CAD build for the part. Positions are in the model's coordinates, mm. A direction names the side the tool comes from. Round coordinates to 2 decimals unless told otherwise and drop trailing zeros. Loops run counter-clockwise (first coordinate to the right, second up) from the corner with the lowest first, then second, coordinate; pieces in that order, holes last.
from build123d import *

# Parameters (mm, degrees)
SKETCH1_R                = 4.25
BOSS_EXTRUDE1_DEPTH      = 4
BOSS_EXTRUDE2_DEPTH      = 4
SKETCH3_R                = 2
BOSS_EXTRUDE3_DEPTH      = 2
BOSS_EXTRUDE4_DEPTH      = 53.7
BOSS_EXTRUDE4_DEPTH_BACK = 4
CUT_EXTRUDE1_DEPTH       = 53.7
BOSS_EXTRUDE5_DEPTH      = 120
CUT_EXTRUDE2_DEPTH       = 120
CUT_EXTRUDE2_DEPTH_BACK  = 120
BOSS_EXTRUDE6_DEPTH      = 53.7
BOSS_EXTRUDE6_DEPTH_BACK = 4
CUT_EXTRUDE3_DEPTH       = 53.7
CUT_EXTRUDE4_DEPTH       = 53.7
SKETCH18_W               = 12.575700543
SKETCH18_H               = 12.198178211
CUT_EXTRUDE9_DEPTH       = 98.7
BOSS_EXTRUDE7_DEPTH      = 20
CUT_EXTRUDE11_DEPTH      = 20
SKETCH22_R               = 3
CUT_EXTRUDE12_DEPTH      = 10
CUT_EXTRUDE13_DEPTH      = 99
CUT_EXTRUDE14_DEPTH      = 99
BOSS_EXTRUDE8_DEPTH      = 12


with BuildPart() as part:
    # Sketch1 → Boss-Extrude1 (new body)
    with BuildSketch(Plane.XY):
        Polygon((0, 10), (0, -15), (-30, -35), (-30, 10), (-15, 25), align=None)
        with Locations((-15, 10)):
            Circle(SKETCH1_R, mode=Mode.SUBTRACT)
    extrude(amount=BOSS_EXTRUDE1_DEPTH)



with BuildPart() as body_2:
    # Sketch2 → Boss-Extrude2 (new body)
    with BuildSketch(Plane.XY.offset(-49.7)):
        Polygon((-30, -35), (-30, 10), (-15, 25), (0, 10), (0, -15), align=None)
    extrude(amount=-BOSS_EXTRUDE2_DEPTH)

    # Sketch3 → Boss-Extrude3 (add)
    with BuildSketch(Plane.XY.offset(-49.7)):
        with Locations((-15, 10)):
            Circle(SKETCH3_R)
    extrude(amount=BOSS_EXTRUDE3_DEPTH)


with BuildPart() as part_1:
    add(part.part)

    add(body_2.part)  # Boss-Extrude4 merges body 2
    # Sketch4 → Boss-Extrude4 (add, two sides: drawn at the far end of the back side and taken through both)
    with BuildSketch(Plane.XY.offset(-49.7).offset(-BOSS_EXTRUDE4_DEPTH_BACK)):
        Polygon((-30, -35), (0, -35), (0, -15), align=None)
    extrude(amount=BOSS_EXTRUDE4_DEPTH + BOSS_EXTRUDE4_DEPTH_BACK)

    # Sketch5 → Cut-Extrude1 (cut)
    with BuildSketch(Plane(origin=(0, 0, 0), x_dir=(0, 0, -1), z_dir=(1, 0, 0))):
        Polygon((24.85, -15), (49.7, -15), (49.7, -35), (0, -35), (0, -15), align=None)
    extrude(amount=-CUT_EXTRUDE1_DEPTH, mode=Mode.SUBTRACT)


with BuildPart() as cut_extrude1_piece_1:
    # of the separate pieces the step leaves, piece 1, a body of its own (cut_extrude1_pieces)
    add(part_1.part.solids().sort_by_distance((-30, -35, -49.7))[0])



with BuildPart() as cut_extrude1_piece_2:
    # of the separate pieces the step leaves, piece 2, a body of its own (cut_extrude1_pieces)
    add(part_1.part.solids().sort_by_distance((0, -35, 0))[0])


with BuildPart() as cut_extrude1_piece_1_1:
    add(cut_extrude1_piece_1.part)

    add(cut_extrude1_piece_2.part)  # Boss-Extrude5 merges Cut-Extrude1 piece 2
    # Sketch6 → Boss-Extrude5 (add)
    with BuildSketch(Plane(origin=(0, 0, 0), x_dir=(0, 0, -1), z_dir=(1, 0, 0))):
        Polygon((0, -35), (-4, -35), (24.85, -46.609657949), (53.7, -35), (49.7, -35), (24.85, -45), align=None)
    extrude(amount=-BOSS_EXTRUDE5_DEPTH)

    # Sketch7 → Cut-Extrude2 (cut, two sides: drawn at the far end of the back side and taken through both)
    with BuildSketch(Plane.XY.offset(-49.7).offset(-CUT_EXTRUDE2_DEPTH_BACK)):
        Polygon((-30, -35), (-120, -35), (-120, -46.609657949), align=None)
    extrude(amount=CUT_EXTRUDE2_DEPTH + CUT_EXTRUDE2_DEPTH_BACK, mode=Mode.SUBTRACT)

    # Sketch8 → Boss-Extrude6 (add, two sides: drawn at the far end of the back side and taken through both)
    with BuildSketch(Plane.XY.offset(-49.7).offset(-BOSS_EXTRUDE6_DEPTH_BACK)):
        Polygon((-30, -35), (-30, -12.5), (-120, -46.609657949), align=None)
    extrude(amount=BOSS_EXTRUDE6_DEPTH + BOSS_EXTRUDE6_DEPTH_BACK)

    # Sketch9 → Cut-Extrude3 (cut)
    with BuildSketch(Plane(origin=(3.949939329, -30.620586856, 0), x_dir=(0.991782404932817, 0.12793616089940293, 0), z_dir=(0.12793616089940293, -0.991782404932817, 0))):
        Polygon((-124.976949291, -24.85), (-34.231237779, -53.7), (-124.976949291, -53.7), align=None)
    extrude(amount=-CUT_EXTRUDE3_DEPTH, mode=Mode.SUBTRACT)

    # Sketch10 → Cut-Extrude4 (cut)
    with BuildSketch(Plane(origin=(3.949939329, -30.620586856, 0), x_dir=(0.991782404932817, 0.12793616089940293, 0), z_dir=(0.12793616089940293, -0.991782404932817, 0))):
        Polygon((-124.976949291, -24.85), (-34.231237779, 4), (-124.976949291, 4), align=None)
    extrude(amount=-CUT_EXTRUDE4_DEPTH, mode=Mode.SUBTRACT)

    # Sketch18 → Cut-Extrude9 (cut)
    with BuildSketch(Plane(origin=(-100, 0, 0), x_dir=(0, 0, -1), z_dir=(1, 0, 0))):
        with Locations((24.80300407, -45.072632523)):
            Rectangle(SKETCH18_W, SKETCH18_H)
    extrude(amount=-CUT_EXTRUDE9_DEPTH, mode=Mode.SUBTRACT)

    # Sketch19 → Boss-Extrude7 (add)
    with BuildSketch(Plane.ZY.offset(100)):
        Polygon((-31.090854341, -39.02973396), (-31.090854341, -44.098247751), (-24.85, -46.609657949), (-18.515153798, -44.060424064), (-18.515153798, -39.02973396), align=None)
    extrude(amount=BOSS_EXTRUDE7_DEPTH)

    # Sketch20 → Cut-Extrude11 (cut)
    with BuildSketch(Plane.ZY.offset(120)):
        with BuildLine():
            Line((-18.515153798, -39.02973396), (-24.80300407, -39.02973396))
            Line((-24.80300407, -39.02973396), (-24.804747468, -39.310924888))
            ThreePointArc((-24.804747468, -39.310924888), (-22.337699017, -40.346275812), (-21.317663529, -42.819695955))
            ThreePointArc((-21.317663529, -42.819695955), (-21.889089638, -44.738955206), (-23.417250653, -46.033098856))
            Line((-23.417250653, -46.033098856), (-18.515153798, -44.060424064))
            Line((-18.515153798, -44.060424064), (-18.515153798, -39.02973396))
        make_face()
        with BuildLine():
            Line((-24.804747468, -39.310924888), (-24.80300407, -39.02973396))
            Line((-24.80300407, -39.02973396), (-31.090854341, -39.02973396))
            Line((-31.090854341, -39.02973396), (-31.090854341, -44.098247751))
            Line((-31.090854341, -44.098247751), (-24.85, -46.609657949))
            Line((-24.85, -46.609657949), (-24.848256601, -46.328467021))
            ThreePointArc((-24.848256601, -46.328467021), (-28.335273102, -42.797941388), (-24.804747468, -39.310924888))
        make_face()
        with BuildLine():
            ThreePointArc((-23.617143522, -46.113538642), (-24.223054162, -46.276254695), (-24.848256601, -46.328467021))
            Line((-24.848256601, -46.328467021), (-24.85, -46.609657949))
            Line((-24.85, -46.609657949), (-23.617143522, -46.113538642))
        make_face()
    extrude(amount=-CUT_EXTRUDE11_DEPTH, mode=Mode.SUBTRACT)

    # Sketch22 → Cut-Extrude12 (cut)
    with BuildSketch(Plane.ZY.offset(120)):
        with Locations((-24.826502035, -42.819695955)):
            Circle(SKETCH22_R)
    extrude(amount=-CUT_EXTRUDE12_DEPTH, mode=Mode.SUBTRACT)

    # Sketch23 → Cut-Extrude13 (cut)
    with BuildSketch(Plane(origin=(-30, 0, 0), x_dir=(0, 0, -1), z_dir=(1, 0, 0))):
        Polygon((0, -12.5), (24.300610602, -23.722317099), (49.7, -12.5), align=None)
    extrude(amount=-CUT_EXTRUDE13_DEPTH, mode=Mode.SUBTRACT)

    # Sketch24 → Cut-Extrude14 (cut)
    with BuildSketch(Plane(origin=(-30, 0, 0), x_dir=(0, 0, -1), z_dir=(1, 0, 0))):
        Polygon((0, -12.5), (24.85, -35), (49.7, -12.5), (24.300610602, -23.722317099), align=None)
    extrude(amount=-CUT_EXTRUDE14_DEPTH, mode=Mode.SUBTRACT)

    # Sketch25 → Boss-Extrude8 (add)
    with BuildSketch(Plane(origin=(-30, 0, 0), x_dir=(0, 0, -1), z_dir=(1, 0, 0))):
        Polygon((0, -35), (49.7, -35), (24.85, -45), align=None)
    extrude(amount=-BOSS_EXTRUDE8_DEPTH)


solid = cut_extrude1_piece_1_1.part
Item 1: Cut at A-A (y = 0.5). List the corners of the cut face in (x, z), plus the area to 3 significant figures.
Verdict:
outline: (-30, -53.7) - (0, -53.7) - (0, -49.7) - (-30, -49.7) - close; (-30, 0) - (0, 0) - (0, 4) - (-30, 4) - close
area: 240 mm2
Item 2: Mould opens along Y. For faces 1 (the flat face through (-42, -40, -25)), 2 (the flat face through (-58.98, -30.41, -44.75)), 3 (the flat face through (-70.668, -27.913, -16.436)) say: released by +Y, released by -Y, zero draft, split by the parting line, or undercut.
Verdict:
face 1: undercut
face 2: released by -Y
face 3: released by +Y
Item 3: Cut at C-C (x = -76). List the corners of the cut face in (y, z), plus the area to 3 significant figures.
Verdict:
outline: (-46.61, -24.85) - (-40.93, -38.95) - (-29.93, -39.4) - (-29.93, -30.45) - (-35, -24.85) - (-29.93, -19.25) - (-29.93, -10.3) - (-40.93, -10.75) - close; hole (-45, -24.85) - (-40.93, -34.95) - (-40.93, -14.75) - close
area: 326 mm2
Item 4: Cut at D-D (x = -62). List the corners of the cut face in (y, z).
Verdict:
outline: (-46.61, -24.85) - (-39.13, -43.44) - (-24.63, -44.03) - (-24.63, -36.31) - (-35, -24.85) - (-24.63, -13.39) - (-24.63, -5.67) - (-39.13, -6.26) - close; hole (-45, -24.85) - (-39.13, -39.44) - (-39.13, -10.26) - close
Item 5: Cut at B-B (z = -32.5). List the corners of the cut face in (x, y).
Verdict:
outline: (-96.87, -37.84) - (-96.14, -43.53) - (0, -43.53) - (0, -41.92) - (-30, -41.92) - (-30, -28.07) - (-71.09, -28.07) - close; hole (-83.66, -41.92) - (-42, -41.92) - (-42, -36.55) - close
Item 6: 3-axis set-ups, long thin cutter, end or side, ignore diameter. For faces 4 (the cylindrical face through (-115.07, -43.969, -22.055)), 5 (the cylindrical face through (-15, 12, -49)), 6 (the flat face through (-46.08, -28.59, -17.77)), 7 (the flat face through (-30, -1, -52)), 8 (the flat face through (-15, 10, -47.7)): which of +Z, -Z, +X, -X, +Y, -Y reach the whole face in a straight line?
Verdict:
face 4: -X
face 5: +Z
face 6: +X, -X, +Y
face 7: +Z, -Z, -X, +Y
face 8: +Z, +X, -X, +Y
Item 7: Flat gauge pins, fed straight in: P1, Ø2, axis at y = 2, z = 2, coming from the -X side; P2, Ø4, axis at x = -68.5, z = -28, coming from the -Y side; P3, Ø6, axis at y = -28, z = -20.5, coming from the +X side; P4, Ø5, axis at x = -49.5, y = -17, coming from the -Z side. Where does each tip first touch, or does it go through?
Verdict:
P1: stops at x = -30
P2: stops at y = -46.15
P3: stops at x = -30
P4: passes through
Item 8: Wall check: L1, parallel to Z at x = -25, y = -34; L2, parallel to Z at x = -33.5, y = -31.5; L3, parallel to X at y = -8.5, z = 1.5. Give the ranges that are in metal, low to high.
Verdict:
L1: z = -53.7 to -49.7, 0 to 4
L2: z = -52.74 to -28.72, -20.98 to 3.04
L3: x = -30 to 0
